Print and shaded views of the part. All mm, measured from the part's lowest x, y and z. Round coordinates to 2 decimals unless told otherwise and drop trailing zeros. Order: outer loops, then holes, each group sorted by start corner. A loop starts at its lowest first (then second) coordinate and runs counter-clockwise, first axis right, second up. Notation, with made-up numbers: M 82,87 L 129,87 A8 ccw 129,92 Z; hole C -34,-15 d8. An arc over 180 degrees is marked long. Write each question's results on one line, items separated by ' | '. Start each with the question number.
1. Two-plate mould, pull along Y, no slides. Class the marked faces 1, 2 and 3: +Y half, -Y half, draft (parallel to the pull), parting line (faces both ways), or undercut.
2. Band-saw the part on D-D, the plane z = 3. List the corners of the cut face in (x, y) (1 decimal).
3. Probe L1, parallel to X at y = 18, z = 27 (1 decimal); L2, parallel to Y at x = 25, z = 20 (1 decimal); L3, parallel to Y at x = 19, z = 31.5 (1 decimal). List the from-to ranges inside material, lowest first. Write a range as [from, to].
4. Band-saw the part on C-C, the plane z = 37. List the corners of the cut face in (x, y) (1 decimal).
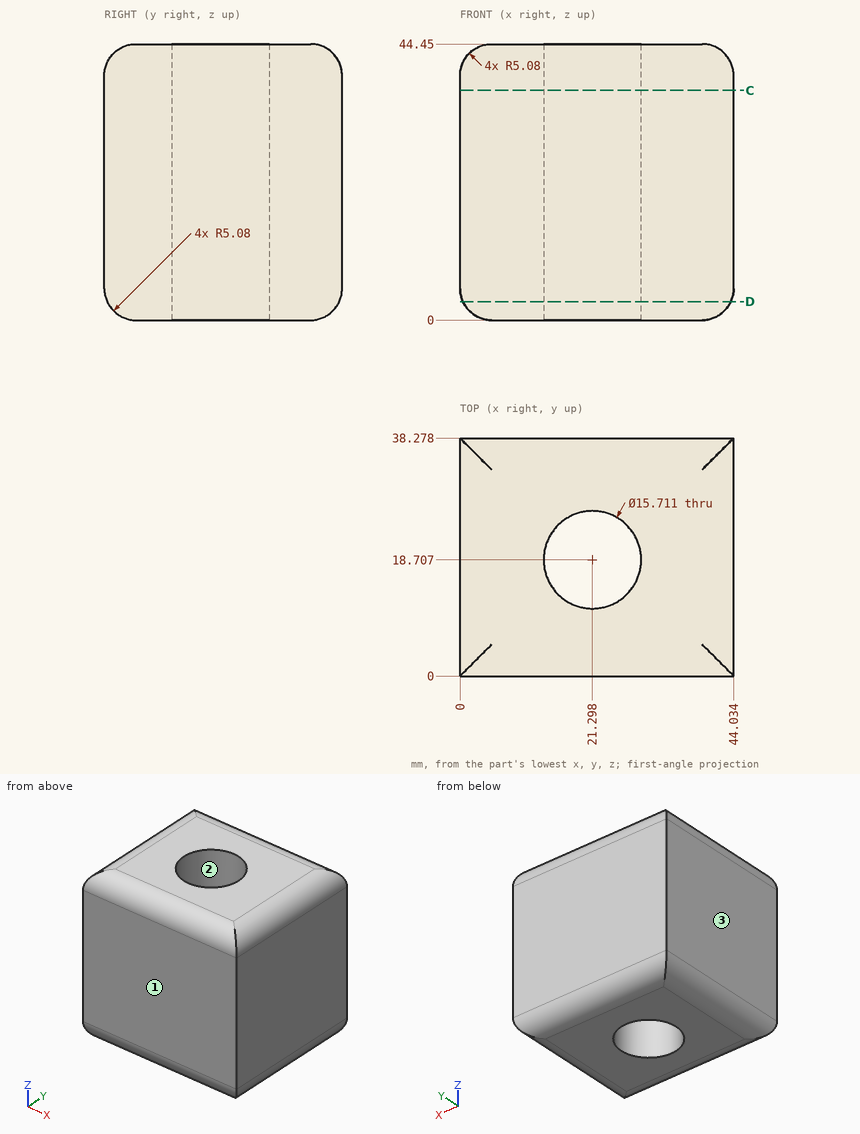
Solution:
1) face 1: -Y half | face 2: undercut | face 3: draft
2) outline: M 0.4,0.4 L 43.6,0.4 L 43.6,37.8 L 0.4,37.8 Z; hole C 21.3,18.7 d15.7
3) L1: [0, 13.5], [29.1, 44] | L2: [0, 11.8], [25.6, 38.3] | L3: [0, 11.2], [26.2, 38.3]
4) outline: M 0,0 L 44,0 L 44,38.3 L 0,38.3 Z; hole C 21.3,18.7 d15.7
